from build123d import *

# Parameters (mm, degrees)
SKETCH1_W           = 76.2
SKETCH1_H           = 101.6
BOSS_EXTRUDE1_DEPTH = 6.35
SKETCH2_R           = 1.7
CUT_EXTRUDE1_DEPTH  = 218.110576665
CUT_EXTRUDE2_DEPTH  = 218.110576665
BOSS_EXTRUDE2_DEPTH = 50.8
BOSS_EXTRUDE5_START = 19.05
SKETCH8_W           = 203.2
SKETCH8_H           = 12.7
SKETCH8_R           = 1.7
BOSS_EXTRUDE5_DEPTH = 19.05


with BuildPart() as part:
    # Sketch1 → Boss-Extrude1 (new body)
    with BuildSketch(Plane(origin=(0, 0, 0), x_dir=(1, 0, 0), z_dir=(0, 1, 0))):
        with Locations((38.1, 50.8)):
            Rectangle(SKETCH1_W, SKETCH1_H)
        with Locations((38.1, 152.4)):
            Rectangle(SKETCH1_W, SKETCH1_H)
    extrude(amount=BOSS_EXTRUDE1_DEPTH)

    # Sketch2 → Cut-Extrude1 (cut, through all)
    with BuildSketch(Plane(origin=(0, 6.35, 0), x_dir=(1, 0, 0), z_dir=(0, 1, 0))):
        with Locations(Location((5, 96.6, 0), (0, 0, 270))):
            Circle(SKETCH2_R)
        with Locations(Location((71.2, 96.6, 0), (0, 0, 270))):
            Circle(SKETCH2_R)
        with Locations(Location((5, 5, 0), (0, 0, 270))):
            Circle(SKETCH2_R)
        with Locations(Location((71.2, 5, 0), (0, 0, 270))):
            Circle(SKETCH2_R)
        with Locations(Location((71.12, 198.12, 0), (0, 0, 270))):
            Circle(SKETCH2_R)
    extrude(amount=-CUT_EXTRUDE1_DEPTH, mode=Mode.SUBTRACT)

    # Sketch3 → Cut-Extrude2 (cut, through all)
    with BuildSketch(Plane.ZY):
        Polygon((-20, 6.35), (0, 3.175), (0, 6.35), align=None)
    extrude(amount=-CUT_EXTRUDE2_DEPTH, mode=Mode.SUBTRACT)


with BuildPart() as body_2:
    # Mirror3: mirrored copy
    add(part.part.mirror(Plane.ZY.offset(25.4)))


with BuildPart() as part_1:
    add(part.part)

    add(body_2.part)  # Boss-Extrude2 merges body 2
    # Sketch5 → Boss-Extrude2 (add)
    with BuildSketch(Plane(origin=(-50.8, 0, 0), x_dir=(0, 0, -1), z_dir=(1, 0, 0))):
        Polygon((20, 6.35), (203.2, 6.35), (203.2, 0), (0, 0), (0, 3.175), align=None)
    extrude(amount=BOSS_EXTRUDE2_DEPTH)

    # Sketch8 → Boss-Extrude5 (add)
    with BuildSketch(Plane(origin=(0, 6.35, 0), x_dir=(1, 0, 0), z_dir=(0, 1, 0)).offset(BOSS_EXTRUDE5_START)):
        with Locations((-25.4, 196.85)):
            Rectangle(SKETCH8_W, SKETCH8_H)
        with Locations(Location((-121.92, 198.12, 0), (0, 0, 270))):
            Circle(SKETCH8_R, mode=Mode.SUBTRACT)
        with Locations(Location((71.12, 198.12, 0), (0, 0, 270))):
            Circle(SKETCH8_R, mode=Mode.SUBTRACT)
    extrude(amount=-BOSS_EXTRUDE5_DEPTH)


solid = part_1.part
Part model, mm, in its own coordinate system. A direction names the side the tool comes from. Give positions to 0.01 mm unless a question says otherwise; leave off trailing zeros. Order: outer loops, then holes, each group sorted by start corner. A loop starts at its lowest first (then second) coordinate and runs counter-clockwise, first axis right, second up. Notation, with made-up numbers: (52.25, 33) -> (60.25, 33) arc R16 cw to (60.25, 61) -> close; hole circle Ø7 at (13, 79.25). An arc over 180 degrees is marked (long way). Use one line per item in the form item = value.
(1) Flat gauge pins, fed straight in: P1, Ø4.5, axis at x = -55.8, z = -5, coming from the +Y side; P2, Ø5.5, axis at x = -42.5, y = 15, coming from the +Z side. Where does each tip first touch, or does it go through?
Solution:
P1 = 4.33
P2 = -190.5
(2) Drill centre lines: line 1 (X direction, y = 3.25, z = -96.6); line 2 (Z direction, x = -55.8, y = 2.6); line 3 (X direction, y = 20, z = -198.12). Where is each one in solid material? Low to high. Write a range as from..to.
Solution:
line_1 = -127..-123.7, -120.3..-57.5, -54.1..3.3, 6.7..69.5, 72.9..76.2
line_2 = -203.2..-98.3, -94.9..-6.7, -3.3..0
line_3 = -127..-123.62, -120.22..69.42, 72.82..76.2
(3) Saw through at B-B (y = 21.25). Write the cut outline in (x, z), then the cut area to 3 significant figures.
Solution:
outline = (-127, -203.2) -> (76.2, -203.2) -> (76.2, -190.5) -> (-127, -190.5) -> close; hole circle Ø3.4 at (-121.92, -198.12); hole circle Ø3.4 at (71.12, -198.12)
area = 2,560 mm²
(4) Saw through at A-A (x = -5). Write the cut outline in (y, z) (3 decimals).
Solution:
outline = (0, -203.2) -> (25.4, -203.2) -> (25.4, -190.5) -> (6.35, -190.5) -> (6.35, -20) -> (3.175, 0) -> (0, 0) -> close
(5) Tool access for faces 1 (the face through (-27, 0, -103)), 2 (the face through (-27, 6.35, -104)): list every direction of +Z, -Z, +X, -X, +Y, -Y with a clear straight run to the whole face (end or side of a thin tool).
Solution:
face_1 = +Z, -Z, +X, -X, -Y
face_2 = +Z, +X, -X, +Y
(6) Saw through at C-C (z = -74.5). Write the cut outline in (x, y).
Solution:
outline = (-127, 0) -> (76.2, 0) -> (76.2, 6.35) -> (-127, 6.35) -> close
